The model under review builds one solid part; all positions refer to its coordinate system, in mm. A direction names the side the tool comes from. Coordinates: 2 decimals unless noted, no trailing zeros. Order: outer loops, then holes, each group sorted by start corner. A loop starts at its lowest first (then second) coordinate and runs counter-clockwise, first axis right, second up. Notation, with made-up numbers: M -34.75,59 L -8.75,59 A18 cw -8.75,85 Z; hole C -30,54.5 d10. An arc over 180 degrees is marked long. Write each question's results on one line, items separated by ' | '.
from build123d import *

# Parameters (mm, degrees)
SKETCH1_R           = 17.5
SKETCH1_R_2         = 5
BOSS_EXTRUDE1_DEPTH = 14.5
SKETCH2_R           = 12.75
SKETCH2_R_2         = 5
BOSS_EXTRUDE2_DEPTH = 8
SKETCH3_R           = 19
SKETCH3_R_2         = 17.5
BOSS_EXTRUDE3_DEPTH = 2
BOSS_EXTRUDE5_START = -14.5
SKETCH3_2_R         = 19
SKETCH3_2_R_2       = 17.5
BOSS_EXTRUDE5_DEPTH = 2


with BuildPart() as part:
    # Sketch1 → Boss-Extrude1 (new body)
    with BuildSketch(Plane.XY):
        Circle(SKETCH1_R)
        Circle(SKETCH1_R_2, mode=Mode.SUBTRACT)
    extrude(amount=BOSS_EXTRUDE1_DEPTH)

    # Sketch2 → Boss-Extrude2 (add)
    with BuildSketch(Plane.XY.offset(14.5)):
        Circle(SKETCH2_R)
        Circle(SKETCH2_R_2, mode=Mode.SUBTRACT)
    extrude(amount=BOSS_EXTRUDE2_DEPTH)

    # Sketch3 → Boss-Extrude3 (add)
    with BuildSketch(Plane(origin=(0, 0, 0), x_dir=(-1, 0, 0), z_dir=(0, 0, -1))):
        Circle(SKETCH3_R)
        Circle(SKETCH3_R_2, mode=Mode.SUBTRACT)
    extrude(amount=-BOSS_EXTRUDE3_DEPTH)

    # Sketch3<2> → Boss-Extrude5 (add)
    with BuildSketch(Plane(origin=(0, 0, 0), x_dir=(-1, 0, 0), z_dir=(0, 0, -1)).offset(BOSS_EXTRUDE5_START)):
        Circle(SKETCH3_2_R)
        Circle(SKETCH3_2_R_2, mode=Mode.SUBTRACT)
    extrude(amount=BOSS_EXTRUDE5_DEPTH)


solid = part.part
1) For faces 1 (the flat face through (-6, -17, 12.5)), 2 (the flat face through (-12.4, -4, 14.5)), 3 (the flat face through (5.5, 0.2, 22.5)), list the 3-axis set-ups (+Z, -Z, +X, -X, +Y, -Y) from which the entire face can be reached by the end or side of a thin tool; tool diameter is ignored.
Solutions:
face 1: none | face 2: +Z | face 3: +Z, +X, -X, +Y, -Y
2) Take a section at A-A on x = 0. State the section outline as (y, z) points, plus the area to 4 significant figures.
Solutions:
outline: M -19,0 L -5,0 L -5,22.5 L -12.75,22.5 L -12.75,14.5 L -19,14.5 L -19,12.5 L -17.5,12.5 L -17.5,2 L -19,2 Z; M 5,0 L 19,0 L 19,2 L 17.5,2 L 17.5,12.5 L 19,12.5 L 19,14.5 L 12.75,14.5 L 12.75,22.5 L 5,22.5 Z | area: 498.5 mm2
3) The part is to be moulded in two halves that separate along Z. For faces 4 (the flat face through (-4, -4, 0)), 5 (the cylindrical face through (-8.767, -16.856, 0.986)), 6 (the flat face through (-6, -17, 2)), say which applies: pulls with the +Z half, pulls with the -Z half, needs draft (parallel to the pull), parting line crosses it, or undercut.
Solutions:
face 4: pulls with the -Z half | face 5: needs draft | face 6: undercut
4) Take a section at C-C on z = 8. State the section outline as (x, y) points.
Solutions:
outline: C 0,0 d35; hole C 0,0 d10
5) To check wall thickness, follow line 1 along Z through (x, y) = (-9, -15.5); line 2 along Y through (x, z) = (0, 8); line 3 along Y through (x, z) = (0, 13). State the ranges of each line that lie inside material, in increasing order.
Solutions:
line 1: 0 to 2, 12.5 to 14.5 | line 2: -17.5 to -5, 5 to 17.5 | line 3: -19 to -5, 5 to 19
6) For pin 1 (4 mm diameter, centred on x = 3.5, z = 17.5, fed in from +Y); pin 2 (1 mm diameter, centred on y = -13.5, z = 7, fed in from -X); pin 3 (1.5 mm diameter, centred on x = 14.5, z = 8.5, fed in from -Y), all flat-tipped, find the tip position at first contact; note any pin that passes through.
Solutions:
pin 1: y = 12.66 | pin 2: x = -11.72 | pin 3: y = -10.83
7) Take a section at D-D on x = -16.5. State the section outline as (y, z) points, plus the area to 3 significant figures.
Solutions:
outline: M -9.42,0 L 9.42,0 L 9.42,2 L 5.83,2 L 5.83,12.5 L 9.42,12.5 L 9.42,14.5 L -9.42,14.5 L -9.42,12.5 L -5.83,12.5 L -5.83,2 L -9.42,2 Z | area: 198 mm2
